Input: dimensioned drawing with shaded views. Units: mm. Origin: part minimum x, y, z. A direction names the side the tool comes from. Round coordinates to 2 decimals unless told otherwise and drop trailing zeros. Loops run counter-clockwise (first coordinate to the right, second up) from the corner with the lowest first, then second, coordinate; pieces in that order, holes last. Notation, with made-up numbers: (46.25, 35.5) - (54.25, 35.5) arc R17 cw to (54.25, 61.5) - close; hole circle Ø7 at (7.5, 60). An arc over 180 degrees is marked (long way). One line per question, with ' | ' between items. Start each with the question number.
Item 1: Draft query along Z for the marked faces 4, 5 and 6. Return one class per face: pulls with the +Z half, pulls with the -Z half, needs draft (parallel to the pull), parting line crosses it, or undercut.
Item 2: First-contact query: pin 1 (2.5 mm diameter, centred on x = 9.5, z = 3.75, fed in from -Y); pin 2 (3.5 mm diameter, centred on x = 6.5, y = 20, fed in from +Z). Flat tips, straight axial feed; report the tip coordinate or a pass-through.
Item 3: Material intervals for line 1 along Z through (x, y) = (3.5, 3.5); line 2 along Y through (x, z) = (6.5, 5.75); line 3 along Z through (x, y) = (1, 26), sorted ascending.
Item 4: Section A-A, the plane x = 6.5. Return loops of the section in (y, z), plus the area to 4 significant figures.
Item 5: Section C-C, the plane y = 20. Return loops of the section in (x, z).
Item 6: Section B-B, the plane y = 6.5. Return loops of the section in (x, z).
Item 7: Section D-D, the plane y = 29.5. Return loops of the section in (x, z), plus the area to 3 significant figures.
Item 8: Set-up query: the marked faces 1, 2 and 3. Return all of +Z, -Z, +X, -X, +Y, -Y with unobstructed straight access to the full face (end or side cutting, diameter ignored); none if empty.
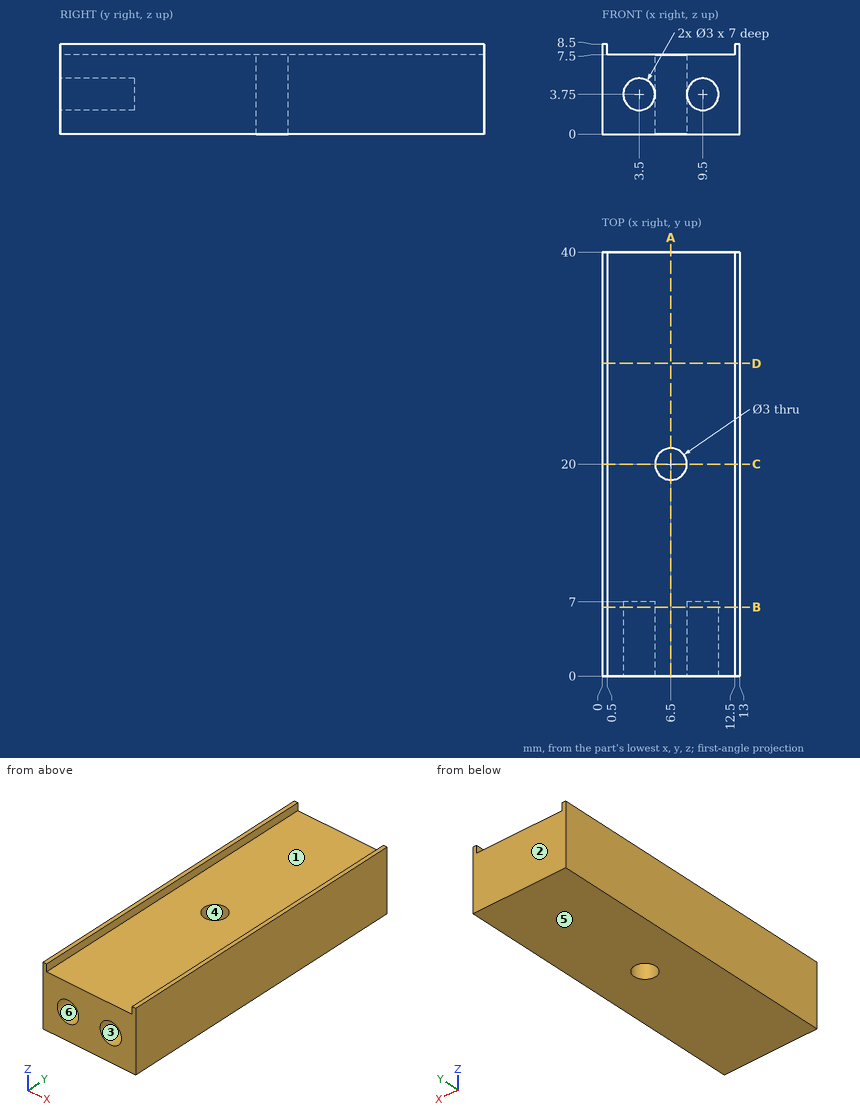
Return value:
1) face 4: needs draft | face 5: pulls with the -Z half | face 6: undercut
2) pin 1: y = 7 | pin 2: z = 7.5
3) line 1: 0 to 2.25, 5.25 to 7.5 | line 2: 0 to 18.5, 21.5 to 40 | line 3: 0 to 7.5
4) outline: (0, 0) - (18.5, 0) - (18.5, 7.5) - (0, 7.5) - close; (21.5, 0) - (40, 0) - (40, 7.5) - (21.5, 7.5) - close | area: 277.5 mm2
5) outline: (0, 0) - (5, 0) - (5, 7.5) - (0.5, 7.5) - (0.5, 8.5) - (0, 8.5) - close; (8, 0) - (13, 0) - (13, 8.5) - (12.5, 8.5) - (12.5, 7.5) - (8, 7.5) - close
6) outline: (0, 0) - (13, 0) - (13, 8.5) - (12.5, 8.5) - (12.5, 7.5) - (0.5, 7.5) - (0.5, 8.5) - (0, 8.5) - close; hole circle Ø3 at (3.5, 3.75); hole circle Ø3 at (9.5, 3.75)
7) outline: (0, 0) - (13, 0) - (13, 8.5) - (12.5, 8.5) - (12.5, 7.5) - (0.5, 7.5) - (0.5, 8.5) - (0, 8.5) - close | area: 98.5 mm2
8) face 1: +Z, +Y, -Y | face 2: +Z, -Z, +X, -X, +Y | face 3: -Y
